```python
from build123d import *

# Parameters (mm, degrees)
SKETCH1_R           = 1.3462
SKETCH1_W           = 5.4034
SKETCH1_H           = 22.6066
SKETCH1_W_2         = 60.6932
SKETCH1_H_2         = 7.81
SKETCH1_W_3         = 5.588
SKETCH1_H_3         = 23.368
BOSS_EXTRUDE1_DEPTH = 3.048
SKETCH2_R           = 10.922
SKETCH2_R_2         = 1.4986
CUT_EXTRUDE1_DEPTH  = 72.310891511


with BuildPart() as part:
    # Sketch1 → Boss-Extrude1 (new body)
    with BuildSketch(Plane.XY):
        with BuildLine():
            Line((57.404932375, 30.507694304), (-34.084892625, 30.507694304))
            ThreePointArc((-34.084892625, 30.507694304), (-36.778969461, 29.391771141), (-37.894892625, 26.697694304))
            Line((-37.894892625, 26.697694304), (-37.894892625, -32.641005696))
            ThreePointArc((-37.894892625, -32.641005696), (-36.778969461, -35.335082532), (-34.084892625, -36.451005696))
            Line((-34.084892625, -36.451005696), (-23.844892625, -33.084405696))
            Line((-23.844892625, -33.084405696), (28.474307375, -33.084405696))
            Line((28.474307375, -33.084405696), (38.714307375, -36.451005696))
            Line((38.714307375, -36.451005696), (57.405007375, -36.451005696))
            ThreePointArc((57.405007375, -36.451005696), (60.108826144, -35.325305244), (61.214907375, -32.613401529))
            Line((61.214907375, -32.613401529), (61.214907375, -28.627805696))
            Line((61.214907375, -28.627805696), (35.575007375, -28.627805696))
            Line((35.575007375, -28.627805696), (35.575007375, -12.628005696))
            Line((35.575007375, -12.628005696), (56.975007375, -12.628005696))
            Line((56.975007375, -12.628005696), (56.975007375, -9.121805696))
            Line((56.975007375, -9.121805696), (40.325007375, -9.121805696))
            Line((40.325007375, -9.121805696), (40.325007375, 4.997894304))
            Line((40.325007375, 4.997894304), (56.975007375, 4.997894304))
            Line((56.975007375, 4.997894304), (56.975007375, 8.658194304))
            Line((56.975007375, 8.658194304), (40.325007375, 8.658194304))
            Line((40.325007375, 8.658194304), (40.325007375, 24.068294304))
            Line((40.325007375, 24.068294304), (61.214907375, 24.068294304))
            Line((61.214907375, 24.068294304), (61.214907375, 26.683892153))
            ThreePointArc((61.214907375, 26.683892153), (60.103884597, 29.386886916), (57.404932375, 30.507694304))
        make_face()
        with Locations(Location((57.405007375, -32.641005696, 0), (0, 0, 180))):
            Circle(SKETCH1_R, mode=Mode.SUBTRACT)
        with Locations(Location((-34.084892625, -32.641005696, 0), (0, 0, 180))):
            Circle(SKETCH1_R, mode=Mode.SUBTRACT)
        with Locations(Location((-34.084892625, 26.697694304, 0), (0, 0, 180))):
            Circle(SKETCH1_R, mode=Mode.SUBTRACT)
        with Locations(Location((57.404932375, 26.697694304, 0), (0, 0, 180))):
            Circle(SKETCH1_R, mode=Mode.SUBTRACT)
        with Locations((16.546707375, -19.663505696)):
            Rectangle(SKETCH1_W, SKETCH1_H, mode=Mode.SUBTRACT)
        with Locations((1.341707375, 21.991994304)):
            Rectangle(SKETCH1_W_2, SKETCH1_H_2, mode=Mode.SUBTRACT)
        with Locations((-26.210892625, -1.882805696)):
            Rectangle(SKETCH1_W_3, SKETCH1_H_3, mode=Mode.SUBTRACT)
    extrude(amount=BOSS_EXTRUDE1_DEPTH)

    # Sketch2 → Cut-Extrude1 (cut, through all)
    with BuildSketch(Plane.XY.offset(3.048)):
        with Locations((-0.302892625, -0.480305696)):
            Circle(SKETCH2_R)
        with Locations((-10.285092625, -10.462505696)):
            Circle(SKETCH2_R_2)
        with Locations((-10.285092625, 9.501894304)):
            Circle(SKETCH2_R_2)
        with Locations((9.679307375, -10.462505696)):
            Circle(SKETCH2_R_2)
        with Locations((9.679307375, 9.501894304)):
            Circle(SKETCH2_R_2)
    extrude(amount=-CUT_EXTRUDE1_DEPTH, mode=Mode.SUBTRACT)


solid = part.part
```
Work out the finished part from the listing and answer in its coordinate system (mm). A direction names the side the tool comes from. Give positions to 0.01 mm unless a question says otherwise; leave off trailing zeros. Write each loop counter-clockwise with the first axis right and the second up, starting at its lowest first coordinate (ties: lowest second). Pieces come first, ordered by that corner, then holes.
(1) The part is cut by section B-B on y = 6.5. Write down the section's boundary in (x, z) (3 decimals).
Final values:
outline: (-37.895, 0) - (-29.005, 0) - (-29.005, 3.048) - (-37.895, 3.048) - close; (-23.417, 0) - (-8.703, 0) - (-8.703, 3.048) - (-23.417, 3.048) - close; (8.097, 0) - (56.975, 0) - (56.975, 3.048) - (8.097, 3.048) - close
(2) Straight lines are drawn through the part: line 1 (Y direction, x = 42.5, z = 2.75); line 2 (X direction, y = -12, z = 2.6) (3 decimals); line 3 (X direction, y = -26.5, z = 1.25) (3 decimals). For each, find the intervals that lie inside material, in ascending order.
Final values:
line 1: y = -36.45 to -28.63, -12.63 to -9.12, 5 to 8.66, 24.07 to 30.51
line 2: x = -37.895 to -29.005, -23.417 to 13.845, 19.248 to 56.975
line 3: x = -37.895 to 13.845, 19.248 to 35.575
(3) The part is cut by section D-D on y = -19. Write down the section's boundary in (x, z) (3 decimals), plus the area to 3 significant figures.
Final values:
outline: (-37.895, 0) - (13.845, 0) - (13.845, 3.048) - (-37.895, 3.048) - close; (19.248, 0) - (35.575, 0) - (35.575, 3.048) - (19.248, 3.048) - close
area: 207 mm2
(4) Which of the six approach directions +Z, -Z, +X, -X, +Y, -Y give full straight-line access (tool end or side, diameter ignored) to faces 4 (the flat face through (11, -3, 0)), 5 (the flat face through (1, 25.897, 2)), 6 (the flat face through (49, -9.122, 2))?
Final values:
face 4: -Z, +X, -X, +Y, -Y
face 5: +Z, -Z
face 6: +Z, -Z, +X
(5) The part is cut by section C-C on x = -5.5. Write down the section's boundary in (y, z).
Final values:
outline: (-33.08, 0) - (-10.09, 0) - (-10.09, 3.05) - (-33.08, 3.05) - close; (9.13, 0) - (18.09, 0) - (18.09, 3.05) - (9.13, 3.05) - close; (25.9, 0) - (30.51, 0) - (30.51, 3.05) - (25.9, 3.05) - close
(6) The mould has two halves that part along X. Classify faces 1 (the flat face through (-29.037, -34.791, 1.503)), 2 (the cylindrical face through (-36.75, 29.42, 1.5)), 3 (the flat face through (51, 24.068, 2)): pulls with the +X half, pulls with the -X half, needs draft (parallel to the pull), parting line crosses it, or undercut.
Final values:
face 1: undercut
face 2: pulls with the -X half
face 3: needs draft
(7) The part is cut by section A-A on x = 49. Write down the section's boundary in (y, z), plus the area to 3 significant figures.
Final values:
outline: (-36.45, 0) - (-28.63, 0) - (-28.63, 3.05) - (-36.45, 3.05) - close; (-12.63, 0) - (-9.12, 0) - (-9.12, 3.05) - (-12.63, 3.05) - close; (5, 0) - (8.66, 0) - (8.66, 3.05) - (5, 3.05) - close; (24.07, 0) - (30.51, 0) - (30.51, 3.05) - (24.07, 3.05) - close
area: 65.3 mm2
(8) Flat-ended cylindrical pins translate along their axes: pin 1 Ø0.9 at (x, z) = (-12, 2) entering from -Y; pin 2 Ø0.9 at (x, z) = (-25, 2) entering from -Y; pin 3 Ø0.9 at (y, z) = (-3, 1.5) entering from +X (3 decimals). Find the tip coordinate at first contact, or state that the pin passes through.
Final values:
pin 1: stops at y = -33.08
pin 2: stops at y = -33.61
pin 3: stops at x = 40.325
